Source: three-view drawing plus pictorial views. Frame: mm from the lowest corner of the part. A direction names the side the tool comes from. Round coordinates to 2 decimals unless told otherwise and drop trailing zeros. Loops run counter-clockwise (first coordinate to the right, second up) from the corner with the lowest first, then second, coordinate; pieces in that order, holes last. Notation, with made-up numbers: M 70.25,-19.5 L 87.25,-19.5 A24 cw 87.25,19.5 Z; hole C 61.5,48.5 d1. An arc over 180 degrees is marked long. Return JSON: item names as keys, results as strings. Group by question number.
1) Section B-B (z = 15). Output: boundary loops of the cut face in (x, y) (1 decimal).
2) Material intervals for line 1 (Y direction, x = 94, z = 18); line 2 (Z direction, x = 99.5, y = 87); line 3 (X direction, y = 45.5, z = 13) (1 decimal), sorted ascending. Write a range as from..to.
3) Section D-D (y = 50). Output: boundary loops of the cut face in (x, z) (1 decimal).
4) Contact query for flat-ended pins moving along their axis: P1, Ø10, axis at y = 76.5, z = 11, coming from the -X side; P2, Ø1.5, axis at y = 11.5, z = 15, coming from the -X side; P3, Ø3.5, axis at x = 63, z = 7.5, coming from the -Y side; P4, Ø5.5, axis at y = 92, z = 11, coming from the -X side. Output: stop coordinate, or through.
5) Mould query, pull axis Y, two halves, no side actions, for the marked faces 1, 2 and 3. Classes: +Y half, -Y half, draft (parallel to the pull), parting line (faces both ways), or undercut.
6) Access query for the marked faces 4, 5, 6 and 7. Directions: +Z, -Z, +X, -X, +Y, -Y. A direction counts if a zero-diameter tool reaches every point of the face in a straight line with its end or side. Return the directions, or none.
7) Section A-A (x = 95.5). Output: boundary loops of the cut face in (y, z).
8) Section C-C (y = 91.5). Output: boundary loops of the cut face in (x, z) (1 decimal), plus the area to 3 significant figures.
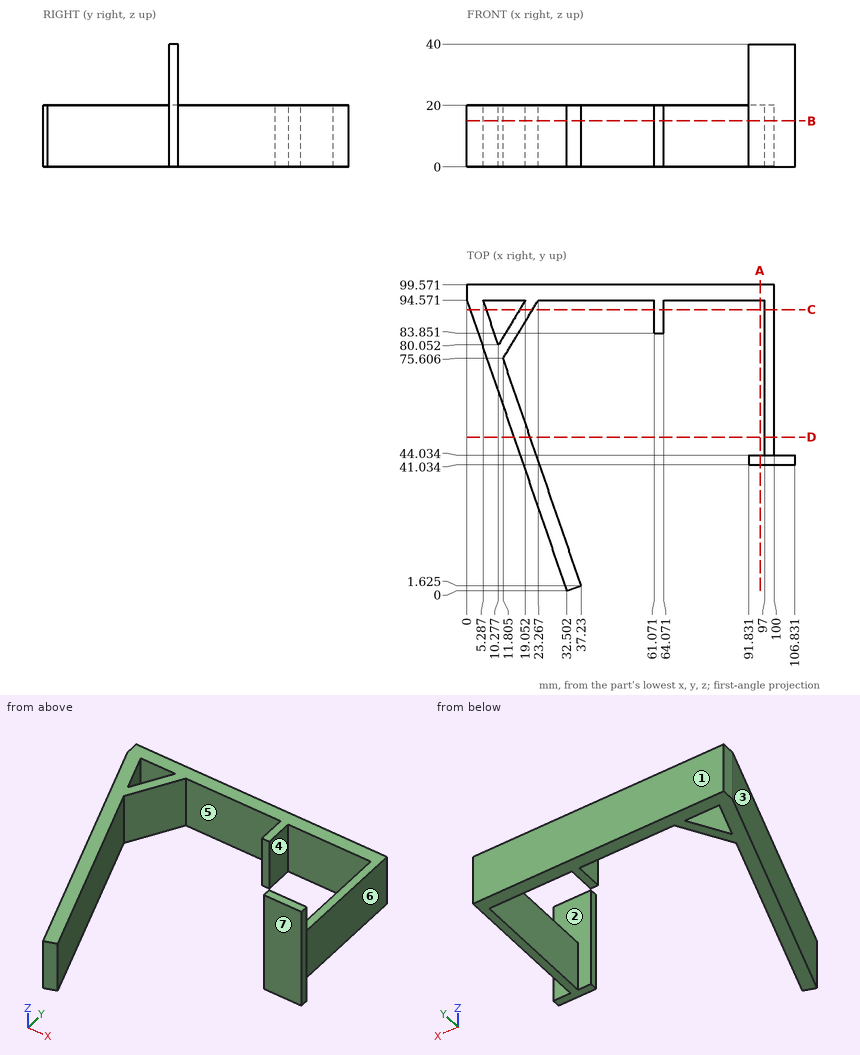
Returned:
{
 "1": {"outline": "M 0,94.6 L 32.5,0 L 37.2,1.6 L 11.8,75.6 L 23.3,94.6 L 61.1,94.6 L 61.1,83.9 L 64.1,83.9 L 64.1,94.6 L 97,94.6 L 97,44 L 91.8,44 L 91.8,41 L 106.8,41 L 106.8,44 L 100,44 L 100,99.6 L 0,99.6 Z; hole M 5.3,94.6 L 10.3,80.1 L 19.1,94.6 Z"},
 "2": {"line 1": "y = 41.03..44.03, 94.57..99.57", "line 2": "z = 0..20", "line 3": "x = 16.9..22.2, 97..100"},
 "3": {"outline": "M 15.3,0 L 20.6,0 L 20.6,20 L 15.3,20 Z; M 97,0 L 100,0 L 100,20 L 97,20 Z"},
 "4": {"P1": "stops at x = 4.49", "P2": "stops at x = 28.29", "P3": "stops at y = 83.85", "P4": "stops at x = 0"},
 "5": {"face 1": "+Y half", "face 2": "undercut", "face 3": "-Y half"},
 "6": {"face 4": "+Z, -Z, -Y", "face 5": "+Z, -Z", "face 6": "+Z, -Z, +X, +Y", "face 7": "+Z, -Z, +X, -Y"},
 "7": {"outline": "M 41.03,0 L 44.03,0 L 44.03,40 L 41.03,40 Z; M 94.57,0 L 99.57,0 L 99.57,20 L 94.57,20 Z"},
 "8": {"outline": "M 1.1,0 L 6.3,0 L 6.3,20 L 1.1,20 Z; M 17.2,0 L 21.4,0 L 21.4,20 L 17.2,20 Z; M 61.1,0 L 64.1,0 L 64.1,20 L 61.1,20 Z; M 97,0 L 100,0 L 100,20 L 97,20 Z", "area": "310 mm^2"}
}
